Geometry check sheet. Reference: the model listing, model coordinates, mm. Coordinates: 2 decimals unless noted, no trailing zeros. Order: outer loops, then holes, each group sorted by start corner. A loop starts at its lowest first (then second) coordinate and runs counter-clockwise, first axis right, second up. Notation, with made-up numbers: (-1.75, -21) - (44.25, -21) arc R22 cw to (44.25, -3) - close; hole circle Ø11 at (34, -28.5). An arc over 180 degrees is marked (long way). Return JSON: item names as keys, results as strings. Group by question number.
Item 1: Section check B-B on y = 0.45. Give the number of separate pieces and of enclosed holes in the cut face, then the cut area to 3 significant figures.
Item 2: Scan lines: probe 1 along Z at (x, y) = (0.55, 0.5); probe 2 along Z at (x, y) = (-42, 0.65); probe 3 along Z at (x, y) = (25, 1.5). Record each from-to range of solid material in increasing order.
Item 3: Gauge pin test, flat end, axial feed: pin 1 (6.5 mm diameter, centred on x = 38.015, z = 0, fed in from +Y). Record the tip position at first contact, or that the pin passes through.
Item 4: Section check A-A on z = 0. Enter the section's corners in (x, y) (3 decimals).
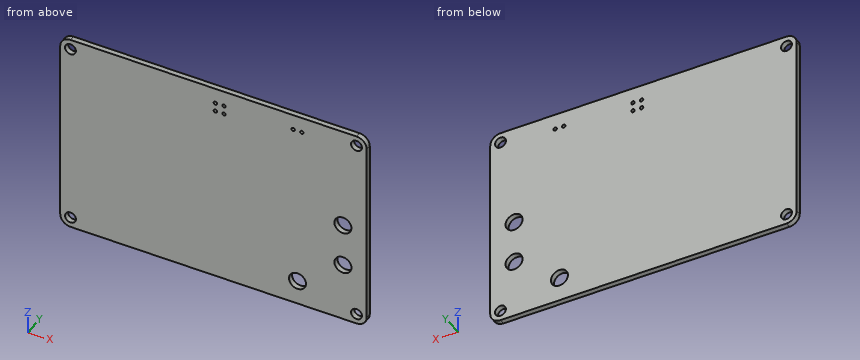
from build123d import *

# Parameters (mm, degrees)
SKETCH1_W           = 90
SKETCH1_H           = 60
BOSS_EXTRUDE1_DEPTH = 1.6
SKETCH2_R           = 1.6
CUT_EXTRUDE1_DEPTH  = 1.6
FILLET1_R           = 3
SKETCH3_R           = 0.5
SKETCH3_R_2         = 2.5
CUT_EXTRUDE2_DEPTH  = 1.6


with BuildPart() as part:
    # Sketch1 → Boss-Extrude1 (new body)
    with BuildSketch(Plane(origin=(0, 0, 0), x_dir=(1, 0, 0), z_dir=(0, 1, 0))):
        Rectangle(SKETCH1_W, SKETCH1_H)
    extrude(amount=BOSS_EXTRUDE1_DEPTH)

    # Sketch2 → Cut-Extrude1 (cut)
    with BuildSketch(Plane(origin=(0, 1.6, 0), x_dir=(-1, 0, 0), z_dir=(0, 1, 0))):
        with Locations((42, -27)):
            Circle(SKETCH2_R)
        with Locations((42, 27)):
            Circle(SKETCH2_R)
        with Locations((-42, 27)):
            Circle(SKETCH2_R)
        with Locations((-42, -27)):
            Circle(SKETCH2_R)
    extrude(amount=-CUT_EXTRUDE1_DEPTH, mode=Mode.SUBTRACT)

    # Fillet1
    fillet1_edges = [part.edges().sort_by_distance(p)[0] for p in [
        (-45, 0.8, -30),
        (45, 0.8, -30),
        (45, 0.8, 30),
        (-45, 0.8, 30),
    ]]
    fillet(fillet1_edges, radius=FILLET1_R)

    # Sketch3 → Cut-Extrude2 (cut)
    with BuildSketch(Plane(origin=(0, 1.6, 0), x_dir=(-1, 0, 0), z_dir=(0, 1, 0))):
        with Locations((-0.55, 25.4)):
            Circle(SKETCH3_R)
        with Locations((-0.55, 22.86)):
            Circle(SKETCH3_R)
        with Locations((-3.09, 25.4)):
            Circle(SKETCH3_R)
        with Locations((-3.09, 22.86)):
            Circle(SKETCH3_R)
        with Locations((-23.41, 25.4)):
            Circle(SKETCH3_R)
        with Locations((-25.95, 25.4)):
            Circle(SKETCH3_R)
        with Locations((-38.015, 0)):
            Circle(SKETCH3_R_2)
        with Locations((-38.015, -12.7)):
            Circle(SKETCH3_R_2)
        with Locations((-24.68, -22.8)):
            Circle(SKETCH3_R_2)
    extrude(amount=-CUT_EXTRUDE2_DEPTH, mode=Mode.SUBTRACT)


solid = part.part
Computed:
{
 "1": {"separate pieces": "1", "enclosed holes": "13", "area": "5,300 mm²"},
 "2": {"probe 1": "z = -30 to 22.36, 23.36 to 24.9, 25.9 to 30", "probe 2": "z = -30 to -28.6, -25.4 to 25.4, 28.6 to 30", "probe 3": "z = -30 to -25.28, -20.32 to 30"},
 "3": {"pin 1": "stops at y = 1.6"},
 "4": {"outline": "(-45, 0) - (35.515, 0) - (35.515, 1.6) - (-45, 1.6) - close; (40.515, 0) - (45, 0) - (45, 1.6) - (40.515, 1.6) - close"}
}
